Read the model definition and answer for the solid it produces. Units are mm, in the model's axes. A direction names the side the tool comes from. Coordinates: 2 decimals unless noted, no trailing zeros. Write each loop counter-clockwise with the first axis right and the second up, starting at its lowest first coordinate (ties: lowest second). Pieces come first, ordered by that corner, then holes. Notation, with made-up numbers: (-22.75, -24) -> (27.25, -24) arc R21 ccw to (27.25, -4) -> close; hole circle Ø1 at (7, 79.5). An arc over 180 degrees is marked (long way). One line per item, written item: value. Start each with the question number.
1. Find section A-A, the plane y = 14.5. Write down the section's boundary in (x, z).
2. Given P1, Ø5, axis at x = -36, y = 2.5, coming from the +Z side; P2, Ø6, axis at x = -0.5, y = -2.5, coming from the +Z side; P3, Ø5, axis at x = -20.5, y = 8.5, coming from the +Z side, each flat-ended and moving along its own axis, determine where each tip first touches the part or whether it passes through.
3. Find section C-C, the plane x = -40. Write down the section's boundary in (y, z), and give its area (3 significant figures).
4. For a pull along Y with two mould halves and no side action, classify faces 6 (the flat face through (-3, -8.087, 1)), 7 (the flat face through (-44, 7, 2)), 8 (the flat face through (-28.876, 7, 2)), 9 (the flat face through (-44, 21.913, 2)) as pulls with the +Y half, pulls with the -Y half, needs draft (parallel to the pull), parting line crosses it, or undercut.
5. Find section D-D, the plane y = 9.5. Write down the section's boundary in (x, z), and give its area (3 significant figures).
6. For faces 1 (the flat face through (-58.876, 7, 2)), 2 (the flat face through (12.124, 7, 1)), 3 (the flat face through (-44, -4.47, 3)), 4 (the flat face through (-13, 7, 3)), 5 (the flat face through (-23, 7, 0.4)), determine the directions among +Z, -Z, +X, -X, +Y, -Y from which every point of the face is accessible in a straight line to the end or side of a thin tool.
7. Find section B-B, the plane z = 1.4. Write down the section's boundary in (x, y), and give its area (3 significant figures).
8. Consider line 1 along X through (y, z) = (9, 2.05); line 2 along X through (y, z) = (1, 1.75); line 3 along Y through (x, z) = (-10.5, 2.7). Determine where each line is inside the solid, lowest interval first.
```python
from build123d import *

# Parameters (mm, degrees)
SKETCH1_W           = 23.094824398
SKETCH1_H           = 22.76684371
SKETCH1_W_2         = 18.65884575
SKETCH1_H_2         = 19.89847104
BOSS_EXTRUDE1_DEPTH = 2
BOSS_EXTRUDE2_DEPTH = 4
BOSS_EXTRUDE3_DEPTH = 3
SKETCH1_5_W         = 11
SKETCH1_5_H         = 10
BOSS_EXTRUDE4_DEPTH = 0.4


with BuildPart() as part:
    # Sketch1 → Boss-Extrude1 (new body)
    with BuildSketch(Plane.XY):
        with Locations((-43.876243767, 6.913043478)):
            Rectangle(SKETCH1_W, SKETCH1_H)
        with Locations((-2.876243767, 6.913043478)):
            Rectangle(SKETCH1_W_2, SKETCH1_H_2)
        Polygon((-55.423655966, 18.296465333), (-32.328831568, 18.296465333), (-28.876243767, 21.913043478), (-58.876243767, 21.913043478), align=None)
        Polygon((-32.328831568, -4.470378377), (-28.876243767, -8.086956522), (-58.876243767, -8.086956522), (-58.876243767, 21.913043478), (-55.423655966, 18.296465333), (-55.423655966, -4.470378377), align=None)
        Polygon((-32.328831568, 18.296465333), (-32.328831568, -4.470378377), (-28.876243767, -8.086956522), (-28.876243767, 1.913043478), (-28.876243767, 11.913043478), (-28.876243767, 21.913043478), align=None)
        Polygon((8.220946061, -4.803958995), (12.123756233, -8.086956522), (-17.876243767, -8.086956522), (-17.876243767, 1.913043478), (-17.876243767, 11.913043478), (-17.876243767, 21.913043478), (-13.973433595, 18.630045951), (-13.973433595, -4.803958995), align=None)
        Polygon((8.220946061, 18.630045951), (8.220946061, -4.803958995), (12.123756233, -8.086956522), (12.123756233, 21.913043478), align=None)
        Polygon((-13.973433595, 18.630045951), (8.220946061, 18.630045951), (12.123756233, 21.913043478), (-17.876243767, 21.913043478), align=None)
        Polygon((8.220946061, -3.036192042), (8.220946061, 18.630045951), (6.453179108, 16.862278998), (6.453179108, -3.036192042), align=None)
        Polygon((6.453179108, 16.862278998), (8.220946061, 18.630045951), (-12.205666642, 18.630045951), (-12.205666642, 16.862278998), align=None)
        Polygon((-12.205666642, 16.862278998), (-13.973433595, 16.862278998), (-13.973433595, -4.803958995), (6.453179108, -4.803958995), (6.453179108, -3.036192042), (-12.205666642, -3.036192042), align=None)
        Polygon((-12.205666642, 16.862278998), (-13.973433595, 18.630045951), (-13.973433595, 16.862278998), align=None)
        Polygon((-12.205666642, 18.630045951), (-13.973433595, 18.630045951), (-12.205666642, 16.862278998), align=None)
        Polygon((6.453179108, -4.803958995), (8.220946061, -4.803958995), (6.453179108, -3.036192042), align=None)
        Polygon((6.453179108, -3.036192042), (8.220946061, -4.803958995), (8.220946061, -3.036192042), align=None)
    extrude(amount=BOSS_EXTRUDE1_DEPTH)

    # Sketch1_3 → Boss-Extrude2 (add)
    with BuildSketch(Plane.XY):
        Polygon((-32.328831568, 18.296465333), (-32.328831568, -4.470378377), (-28.876243767, -8.086956522), (-28.876243767, 1.913043478), (-28.876243767, 11.913043478), (-28.876243767, 21.913043478), align=None)
        Polygon((-55.423655966, 18.296465333), (-32.328831568, 18.296465333), (-28.876243767, 21.913043478), (-58.876243767, 21.913043478), align=None)
        Polygon((-32.328831568, -4.470378377), (-28.876243767, -8.086956522), (-58.876243767, -8.086956522), (-58.876243767, 21.913043478), (-55.423655966, 18.296465333), (-55.423655966, -4.470378377), align=None)
    extrude(amount=BOSS_EXTRUDE2_DEPTH)

    # Sketch1_4 → Boss-Extrude3 (add)
    with BuildSketch(Plane.XY):
        Polygon((6.453179108, 16.862278998), (8.220946061, 18.630045951), (-12.205666642, 18.630045951), (-12.205666642, 16.862278998), align=None)
        Polygon((-12.205666642, 18.630045951), (-13.973433595, 18.630045951), (-12.205666642, 16.862278998), align=None)
        Polygon((-12.205666642, 16.862278998), (-13.973433595, 18.630045951), (-13.973433595, 16.862278998), align=None)
        Polygon((-12.205666642, 16.862278998), (-13.973433595, 16.862278998), (-13.973433595, -4.803958995), (6.453179108, -4.803958995), (6.453179108, -3.036192042), (-12.205666642, -3.036192042), align=None)
        Polygon((8.220946061, -3.036192042), (8.220946061, 18.630045951), (6.453179108, 16.862278998), (6.453179108, -3.036192042), align=None)
        Polygon((6.453179108, -3.036192042), (8.220946061, -4.803958995), (8.220946061, -3.036192042), align=None)
        Polygon((6.453179108, -4.803958995), (8.220946061, -4.803958995), (6.453179108, -3.036192042), align=None)
    extrude(amount=BOSS_EXTRUDE3_DEPTH)

    # Sketch1_5 → Boss-Extrude4 (add)
    with BuildSketch(Plane.XY):
        with Locations((-23.376243767, 6.913043478)):
            Rectangle(SKETCH1_5_W, SKETCH1_5_H)
    extrude(amount=BOSS_EXTRUDE4_DEPTH)


solid = part.part
```
Answer block:
1. outline: (-58.88, 0) -> (-28.88, 0) -> (-28.88, 4) -> (-32.33, 4) -> (-32.33, 2) -> (-55.42, 2) -> (-55.42, 4) -> (-58.88, 4) -> close; (-17.88, 0) -> (12.12, 0) -> (12.12, 2) -> (8.22, 2) -> (8.22, 3) -> (6.45, 3) -> (6.45, 2) -> (-12.21, 2) -> (-12.21, 3) -> (-13.97, 3) -> (-13.97, 2) -> (-17.88, 2) -> close
2. P1: stops at z = 2
2. P2: stops at z = 3
2. P3: stops at z = 0.4
3. outline: (-8.09, 0) -> (21.91, 0) -> (21.91, 4) -> (18.3, 4) -> (18.3, 2) -> (-4.47, 2) -> (-4.47, 4) -> (-8.09, 4) -> close
3. area: 74.5 mm2
4. face 6: pulls with the -Y half
4. face 7: undercut
4. face 8: needs draft
4. face 9: pulls with the +Y half
5. outline: (-58.88, 0) -> (12.12, 0) -> (12.12, 2) -> (8.22, 2) -> (8.22, 3) -> (6.45, 3) -> (6.45, 2) -> (-12.21, 2) -> (-12.21, 3) -> (-13.97, 3) -> (-13.97, 2) -> (-17.88, 2) -> (-17.88, 0.4) -> (-28.88, 0.4) -> (-28.88, 4) -> (-32.33, 4) -> (-32.33, 2) -> (-55.42, 2) -> (-55.42, 4) -> (-58.88, 4) -> close
5. area: 142 mm2
6. face 1: +Z, -Z, -X, +Y, -Y
6. face 2: +Z, -Z, +X, +Y, -Y
6. face 3: +Z
6. face 4: +Z, +X, +Y, -Y
6. face 5: +Z, +Y, -Y
7. outline: (-58.88, -8.09) -> (-28.88, -8.09) -> (-28.88, 21.91) -> (-58.88, 21.91) -> close; (-17.88, -8.09) -> (12.12, -8.09) -> (12.12, 21.91) -> (-17.88, 21.91) -> close
7. area: 1,800 mm2
8. line 1: x = -58.88 to -55.42, -32.33 to -28.88, -13.97 to -12.21, 6.45 to 8.22
8. line 2: x = -58.88 to -28.88, -17.88 to 12.12
8. line 3: y = -4.8 to -3.04, 16.86 to 18.63
